Model file for the job. Use its own axes, mm. A direction names the side the tool comes from. Give positions to 0.01 mm unless a question says otherwise; leave off trailing zeros. Write each loop counter-clockwise with the first axis right and the second up, starting at its lowest first coordinate (ties: lowest second). Pieces come first, ordered by that corner, then holes. Notation, with made-up numbers: (80, 36) - (103, 36) arc R20 cw to (103, 53) - close; hole circle Ø10 at (16.25, -26). An arc over 180 degrees is marked (long way). One line per item, written item: value. Start each with the question number.
(1) Cut at D-D, the plane y = 5. List the corners of the cut face in (x, z).
(2) Mould opens along Z. For faces 3 (the face through (-1.172, -8.923, 4.757)), 4 (the face through (-2, 2, -5.25)), 5 (the face through (-5.65, 4.13, -0.06)) say: pulls with the +Z half, pulls with the -Z half, needs draft (parallel to the pull), parting line crosses it, or undercut.
(3) Cut at B-B, the plane x = 2.75. List the corners of the cut face in (y, z).
(4) Probe L1, parallel to Y at x = 0, z = 2.5; L2, parallel to Y at x = -0.5, z = -2.75; L3, parallel to Y at x = -4.75, z = -4. List the from-to ranges inside material, lowest first.
(5) 3-axis set-ups, long thin cutter, end or side, ignore diameter. For faces 1 (the face through (2, 2, 5.25)), 2 (the face through (7, -2, 4.25)): which of +Z, -Z, +X, -X, +Y, -Y reach the whole face in a straight line?
(6) Drop flat-ended pins along their axis: P1, Ø1.5, axis at x = 4, z = -1.5, coming from the +Y side; P2, Ø1, axis at y = -5, z = -4, coming from the -X side; P3, Ø1, axis at y = -3, z = -3, coming from the +X side. Give the stop position or say it passes through.
(7) Cut at A-A, the plane y = -0.75. List the corners of the cut face in (x, z), and give its area (3 significant figures).
(8) Cut at C-C, the plane x = 0.5. List the corners of the cut face in (y, z), and give its area (3 significant figures).
from build123d import *

# Parameters (mm, degrees)
F3_DEPTH = 8.5


with BuildPart() as f1:
    # F0 (on Front) → F1 (revolve)
    with BuildSketch(Plane.XZ):
        Polygon((9, 5.25), (2.5, 5.25), (2.5, -5.25), (9, -5.25), (9, -4.25), (7, -4.25), (7, 4.25), (9, 4.25), align=None)
    revolve(axis=Axis((0, 0, -3.0081442633), (0, 0, -1)))

    # F2 (on face) → F3 (join)
    with BuildSketch(Plane.XY.offset(-4.25)):
        with BuildLine():
            ThreePointArc((7.267101182, -3.4629092409), (6.7053936496, -2.9334995134), (6.657395615, -2.1631189579))
            ThreePointArc((6.657395615, -2.1631189579), (6.2370456655, -3.1779335057), (5.663118949, -4.114496782))
            ThreePointArc((5.663118949, -4.114496782), (6.3145824491, -3.7005096665), (7.0730473275, -3.8437613743))
            ThreePointArc((7.0730473275, -3.8437613743), (7.1726025197, -3.6546235229), (7.267101182, -3.4629092409))
        make_face()
        with BuildLine():
            ThreePointArc((7.9815217391, -1.0477646338), (7.2837095283, -0.7178432371), (7, 0))
            ThreePointArc((7, 0), (6.9138183844, -1.0950412539), (6.657395615, -2.1631189579))
            ThreePointArc((6.657395615, -2.1631189579), (7.1490451706, -1.5680805373), (7.9146553379, -1.4699424759))
            ThreePointArc((7.9146553379, -1.4699424759), (7.9508911418, -1.2592974436), (7.9815217391, -1.0477646338))
        make_face()
        with BuildLine():
            ThreePointArc((7.9146553379, 1.4699424759), (7.1490451776, 1.5680805334), (6.6573956199, 2.1631189425))
            ThreePointArc((6.6573956199, 2.1631189425), (6.9138183857, 1.0950412459), (7, 0))
            ThreePointArc((7, 0), (7.2837095283, 0.7178432371), (7.9815217391, 1.0477646338))
            ThreePointArc((7.9815217391, 1.0477646338), (7.9508911418, 1.2592974436), (7.9146553379, 1.4699424759))
        make_face()
        with BuildLine():
            ThreePointArc((5.8413261283, -5.5390801639), (5.4707071235, -4.8620044306), (5.663118949, -4.114496782))
            ThreePointArc((5.663118949, -4.114496782), (4.9497474683, -4.9497474683), (4.114496782, -5.663118949))
            ThreePointArc((4.114496782, -5.663118949), (4.8620044306, -5.4707071235), (5.5390801639, -5.8413261283))
            ThreePointArc((5.5390801639, -5.8413261283), (5.6922095886, -5.6922095886), (5.8413261283, -5.5390801639))
        make_face()
        with BuildLine():
            ThreePointArc((3.8437613743, -7.0730473275), (3.7005096665, -6.3145824491), (4.114496782, -5.663118949))
            ThreePointArc((4.114496782, -5.663118949), (3.1779334985, -6.2370456692), (2.1631189425, -6.6573956199))
            ThreePointArc((2.1631189425, -6.6573956199), (2.933499506, -6.7053936461), (3.4629092409, -7.267101182))
            ThreePointArc((3.4629092409, -7.267101182), (3.6546235229, -7.1726025197), (3.8437613743, -7.0730473275))
        make_face()
        with BuildLine():
            ThreePointArc((1.4699424759, -7.9146553379), (1.5680805334, -7.1490451776), (2.1631189425, -6.6573956199))
            ThreePointArc((2.1631189425, -6.6573956199), (1.0950412459, -6.9138183857), (0, -7))
            ThreePointArc((0, -7), (0.7178432371, -7.2837095283), (1.0477646338, -7.9815217391))
            ThreePointArc((1.0477646338, -7.9815217391), (1.2592974436, -7.9508911418), (1.4699424759, -7.9146553379))
        make_face()
        with BuildLine():
            ThreePointArc((0, -7), (-1.0950412668, -6.9138183823), (-2.1631189827, -6.6573956069))
            ThreePointArc((-2.1631189827, -6.6573956069), (-1.5680805436, -7.1490451591), (-1.4699424759, -7.9146553379))
            ThreePointArc((-1.4699424759, -7.9146553379), (-1.2592974436, -7.9508911418), (-1.0477646338, -7.9815217391))
            ThreePointArc((-1.0477646338, -7.9815217391), (-0.7178432371, -7.2837095283), (0, -7))
        make_face()
        with BuildLine():
            ThreePointArc((-2.1631189827, -6.6573956069), (-3.1779335128, -6.2370456619), (-4.1144967738, -5.663118955))
            ThreePointArc((-4.1144967738, -5.663118955), (-3.7005096655, -6.314582454), (-3.8437613743, -7.0730473275))
            ThreePointArc((-3.8437613743, -7.0730473275), (-3.6546235229, -7.1726025197), (-3.4629092409, -7.267101182))
            ThreePointArc((-3.4629092409, -7.267101182), (-2.9334995252, -6.7053936551), (-2.1631189827, -6.6573956069))
        make_face()
        with BuildLine():
            ThreePointArc((-4.1144967738, -5.663118955), (-4.9497474777, -4.9497474589), (-5.6631189706, -4.1144967523))
            ThreePointArc((-5.6631189706, -4.1144967523), (-5.4707071212, -4.8620044124), (-5.8413261283, -5.5390801639))
            ThreePointArc((-5.8413261283, -5.5390801639), (-5.6922095886, -5.6922095886), (-5.5390801639, -5.8413261283))
            ThreePointArc((-5.5390801639, -5.8413261283), (-4.8620044256, -5.4707071229), (-4.1144967738, -5.663118955))
        make_face()
        with BuildLine():
            ThreePointArc((-5.6631189706, -4.1144967523), (-6.2370456738, -3.1779334893), (-6.657395615, -2.1631189579))
            ThreePointArc((-6.657395615, -2.1631189579), (-6.7053936496, -2.9334995134), (-7.267101182, -3.4629092409))
            ThreePointArc((-7.267101182, -3.4629092409), (-7.1726025197, -3.6546235229), (-7.0730473275, -3.8437613743))
            ThreePointArc((-7.0730473275, -3.8437613743), (-6.3145824671, -3.700509663), (-5.6631189706, -4.1144967523))
        make_face()
        with BuildLine():
            ThreePointArc((-6.657395615, -2.1631189579), (-6.9138183853, -1.0950412479), (-7, 1.2e-08))
            ThreePointArc((-7, 1.2e-08), (-7.2837095242, -0.7178432327), (-7.9815217391, -1.0477646338))
            ThreePointArc((-7.9815217391, -1.0477646338), (-7.9508911418, -1.2592974436), (-7.9146553379, -1.4699424759))
            ThreePointArc((-7.9146553379, -1.4699424759), (-7.1490451706, -1.5680805373), (-6.657395615, -2.1631189579))
        make_face()
        with BuildLine():
            ThreePointArc((-7, 1.2e-08), (-6.9138183847, 1.0950412518), (-6.6573956199, 2.1631189425))
            ThreePointArc((-6.6573956199, 2.1631189425), (-7.1490451776, 1.5680805334), (-7.9146553379, 1.4699424759))
            ThreePointArc((-7.9146553379, 1.4699424759), (-7.9508911418, 1.2592974436), (-7.9815217391, 1.0477646338))
            ThreePointArc((-7.9815217391, 1.0477646338), (-7.2837095325, 0.7178432415), (-7, 1.2e-08))
        make_face()
        with BuildLine():
            ThreePointArc((-6.6573956199, 2.1631189425), (-6.2370456751, 3.1779334867), (-5.6631189645, 4.1144967607))
            ThreePointArc((-5.6631189645, 4.1144967607), (-6.314582462, 3.700509664), (-7.0730473275, 3.8437613743))
            ThreePointArc((-7.0730473275, 3.8437613743), (-7.1726025197, 3.6546235229), (-7.267101182, 3.4629092409))
            ThreePointArc((-7.267101182, 3.4629092409), (-6.7053936461, 2.933499506), (-6.6573956199, 2.1631189425))
        make_face()
        with BuildLine():
            ThreePointArc((-5.6631189645, 4.1144967607), (-4.9497474683, 4.9497474683), (-4.1144967607, 5.6631189645))
            ThreePointArc((-4.1144967607, 5.6631189645), (-4.8620044176, 5.4707071219), (-5.5390801639, 5.8413261283))
            ThreePointArc((-5.5390801639, 5.8413261283), (-5.6922095886, 5.6922095886), (-5.8413261283, 5.5390801639))
            ThreePointArc((-5.8413261283, 5.5390801639), (-5.4707071219, 4.8620044176), (-5.6631189645, 4.1144967607))
        make_face()
        with BuildLine():
            ThreePointArc((-4.1144967607, 5.6631189645), (-3.1779334867, 6.2370456751), (-2.1631189425, 6.6573956199))
            ThreePointArc((-2.1631189425, 6.6573956199), (-2.933499506, 6.7053936461), (-3.4629092409, 7.267101182))
            ThreePointArc((-3.4629092409, 7.267101182), (-3.6546235229, 7.1726025197), (-3.8437613743, 7.0730473275))
            ThreePointArc((-3.8437613743, 7.0730473275), (-3.700509664, 6.314582462), (-4.1144967607, 5.6631189645))
        make_face()
        with BuildLine():
            ThreePointArc((-8.7e-09, 7), (-0.7178432403, 7.2837095313), (-1.0477646338, 7.9815217391))
            ThreePointArc((-1.0477646338, 7.9815217391), (-1.2592974436, 7.9508911418), (-1.4699424759, 7.9146553379))
            ThreePointArc((-1.4699424759, 7.9146553379), (-1.5680805334, 7.1490451776), (-2.1631189425, 6.6573956199))
            ThreePointArc((-2.1631189425, 6.6573956199), (-1.0950412502, 6.913818385), (-8.7e-09, 7))
        make_face()
        with BuildLine():
            ThreePointArc((1.0477646338, 7.9815217391), (0.7178432339, 7.2837095254), (-8.7e-09, 7))
            ThreePointArc((-8.7e-09, 7), (1.0950412447, 6.9138183858), (2.1631189486, 6.657395618))
            ThreePointArc((2.1631189486, 6.657395618), (1.568080535, 7.1490451748), (1.4699424759, 7.9146553379))
            ThreePointArc((1.4699424759, 7.9146553379), (1.2592974436, 7.9508911418), (1.0477646338, 7.9815217391))
        make_face()
        with BuildLine():
            ThreePointArc((3.4629092409, 7.267101182), (2.9334995089, 6.7053936475), (2.1631189486, 6.657395618))
            ThreePointArc((2.1631189486, 6.657395618), (3.1779335013, 6.2370456677), (4.114496782, 5.663118949))
            ThreePointArc((4.114496782, 5.663118949), (3.7005096665, 6.3145824491), (3.8437613743, 7.0730473275))
            ThreePointArc((3.8437613743, 7.0730473275), (3.6546235229, 7.1726025197), (3.4629092409, 7.267101182))
        make_face()
        with BuildLine():
            ThreePointArc((5.5390801639, 5.8413261283), (4.8620044306, 5.4707071235), (4.114496782, 5.663118949))
            ThreePointArc((4.114496782, 5.663118949), (4.949747481, 4.9497474556), (5.6631189701, 4.114496753))
            ThreePointArc((5.6631189701, 4.114496753), (5.4707071213, 4.8620044128), (5.8413261283, 5.5390801639))
            ThreePointArc((5.8413261283, 5.5390801639), (5.6922095886, 5.6922095886), (5.5390801639, 5.8413261283))
        make_face()
        with BuildLine():
            ThreePointArc((7.0730473275, 3.8437613743), (6.3145824667, 3.7005096631), (5.6631189701, 4.114496753))
            ThreePointArc((5.6631189701, 4.114496753), (6.2370456773, 3.1779334825), (6.6573956199, 2.1631189425))
            ThreePointArc((6.6573956199, 2.1631189425), (6.7053936461, 2.933499506), (7.267101182, 3.4629092409))
            ThreePointArc((7.267101182, 3.4629092409), (7.1726025197, 3.6546235229), (7.0730473275, 3.8437613743))
        make_face()
    extrude(amount=F3_DEPTH)


solid = f1.part
Answers follow:
1. outline: (-7.48, -5.25) - (7.48, -5.25) - (7.48, -4.25) - (5.5, -4.25) - (5.5, 4.25) - (7.48, 4.25) - (7.48, 5.25) - (-7.48, 5.25) - (-7.48, 4.25) - (-5.5, 4.25) - (-5.5, -4.25) - (-7.48, -4.25) - close
2. face 3: needs draft
2. face 4: pulls with the -Z half
2. face 5: undercut
3. outline: (-8.57, -5.25) - (8.57, -5.25) - (8.57, -4.25) - (6.64, -4.25) - (6.64, 4.25) - (8.57, 4.25) - (8.57, 5.25) - (-8.57, 5.25) - (-8.57, 4.25) - (-6.64, 4.25) - (-6.64, -4.25) - (-8.57, -4.25) - close
4. L1: y = -7 to -2.5, 2.5 to 7
4. L2: y = -7.13 to -2.45, 2.45 to 7.13
4. L3: y = -5.46 to 5.46
5. face 1: +Z, +X, -X, +Y, -Y
5. face 2: none
6. P1: stops at y = 7.27
6. P2: stops at x = -7.76
6. P3: stops at x = 7.27
7. outline: (-8.97, -5.25) - (-2.38, -5.25) - (-2.38, 5.25) - (-8.97, 5.25) - (-8.97, 4.25) - (-7.32, 4.25) - (-7.32, -4.25) - (-8.97, -4.25) - close; (2.38, -5.25) - (8.97, -5.25) - (8.97, -4.25) - (7.32, -4.25) - (7.32, 4.25) - (8.97, 4.25) - (8.97, 5.25) - (2.38, 5.25) - close
7. area: 110 mm²
8. outline: (-8.99, -5.25) - (-2.45, -5.25) - (-2.45, 5.25) - (-8.99, 5.25) - (-8.99, 4.25) - (-7.13, 4.25) - (-7.13, -4.25) - (-8.99, -4.25) - close; (2.45, -5.25) - (8.99, -5.25) - (8.99, -4.25) - (7.13, -4.25) - (7.13, 4.25) - (8.99, 4.25) - (8.99, 5.25) - (2.45, 5.25) - close
8. area: 106 mm²
